```python
from build123d import *

# Parameters (mm, degrees)
F0_W     = 6
F0_H     = 6
F0_R     = 1.75
F2_DEPTH = 3
F1_W     = 9.8
F1_H     = 18
F3_DEPTH = 0.2


with BuildPart() as f2:
    # F0 (on Top) → F2 (new body)
    with BuildSketch(Plane.XY):
        with BuildLine():
            ThreePointArc((1.75, -6), (-1.237437, -4.762563), (0, -7.75))
            ThreePointArc((0, -7.75), (1.237437, -7.237437), (1.75, -6))
        make_face()
        Polygon((7.5, 9), (-7.5, 9), (-7.5, 3), (-7.5, -9), (0, -9), (7.5, -9), (7.5, 3), align=None)
        with BuildLine():
            ThreePointArc((1.75, -6), (1.237437, -7.237437), (0, -7.75))
            ThreePointArc((0, -7.75), (-1.237437, -4.762563), (1.75, -6))
        make_face(mode=Mode.SUBTRACT)
        with BuildLine():
            ThreePointArc((-8.75, 6), (-11.737437, 7.237437), (-10.5, 4.25))
            ThreePointArc((-10.5, 4.25), (-9.262563, 4.762563), (-8.75, 6))
        make_face()
        Polygon((-7.5, 3), (-7.5, 9), (-13.5, 9), (-13.5, 3), (-10.5, 3), align=None)
        with BuildLine():
            ThreePointArc((-8.75, 6), (-9.262563, 4.762563), (-10.5, 4.25))
            ThreePointArc((-10.5, 4.25), (-11.737437, 7.237437), (-8.75, 6))
        make_face(mode=Mode.SUBTRACT)
        with Locations((10.5, 6)):
            Rectangle(F0_W, F0_H)
        with Locations((10.5, 6)):
            Circle(F0_R, mode=Mode.SUBTRACT)
    extrude(amount=F2_DEPTH)

    # F1 (on face) → F3 (cut)
    with BuildSketch(Plane.XY):
        Rectangle(F1_W, F1_H)
    extrude(amount=F3_DEPTH, mode=Mode.SUBTRACT)


solid = f2.part
```
Build history of the part. All positions in model axes, mm. A direction names the side the tool comes from. Coordinates: 2 decimals unless noted, no trailing zeros. Order: outer loops, then holes, each group sorted by start corner. A loop starts at its lowest first (then second) coordinate and runs counter-clockwise, first axis right, second up. Notation, with made-up numbers: M -27,21.5 L 6,21.5 A18 ccw 6,34.5 Z; hole C 89.5,15.25 d11. An arc over 180 degrees is marked long. One line per question, with ' | ' between items. Start each with the question number.
1. Mould opens along Y. For faces 1 (the face through (11.31, 4.45, 1.48)), 2 (the face through (-7, 2, 0)), 3 (the face through (10, 3, 1)) say: +Y half, -Y half, draft (parallel to the pull), parting line (faces both ways), or undercut.
2. Cut at C-C (y = 1.5). Write the cut outline in (x, z), plus the area to 3 significant figures.
3. Cut at B-B (x = 10.5). Write the cut outline in (y, z), plus the area to 3 significant figures.
4. Cut at A-A (z = 2.2). Write the cut outline in (x, y), plus the area to 3 significant figures.
5. Tool access for faces 4 (the face through (0, 0, 0.2)), 5 (the face through (-11, 3, 1)), 6 (the face through (7.5, -3, 1)): list every direction of +Z, -Z, +X, -X, +Y, -Y with a clear straight run to the whole face (end or side of a thin tool).
6. Wall check: line 1 along Y through (x, z) = (10.5, 1.75); line 2 along Y through (x, z) = (0, 1); line 3 along X through (y, z) = (-6, 1.05). Give the ranges that are in metal, low to high. Write a range as [from, to].
7. Flat gauge pins, fed straight in: P1, Ø3, axis at x = -10.5, y = 6, coming from the -Z side; P2, Ø3, axis at x = -1, y = 0.5, coming from the -Z side; P3, Ø1.5, axis at x = -9, z = 2, coming from the -Y side; P4, Ø0.9, axis at y = -3, z = 1.5, coming from the -X side. Where does each tip first touch, or does it go through?
8. Cut at D-D (y = -6.5). Write the cut outline in (x, z).
The answers:
1) face 1: undercut | face 2: draft | face 3: -Y half
2) outline: M -7.5,0 L -4.9,0 L -4.9,0.2 L 4.9,0.2 L 4.9,0 L 7.5,0 L 7.5,3 L -7.5,3 Z | area: 43.0 mm2
3) outline: M 3,0 L 4.25,0 L 4.25,3 L 3,3 Z; M 7.75,0 L 9,0 L 9,3 L 7.75,3 Z | area: 7.50 mm2
4) outline: M -13.5,3 L -7.5,3 L -7.5,-9 L 7.5,-9 L 7.5,3 L 13.5,3 L 13.5,9 L -13.5,9 Z; hole C -10.5,6 d3.5; hole C 0,-6 d3.5; hole C 10.5,6 d3.5 | area: 313 mm2
5) face 4: -Z, +Y, -Y | face 5: +Z, -Z, -X, -Y | face 6: +Z, -Z, +X, -Y
6) line 1: y = [3, 4.25], [7.75, 9] | line 2: y = [-9, -7.75], [-4.25, 9] | line 3: x = [-7.5, -1.75], [1.75, 7.5]
7) P1: passes through | P2: stops at z = 0.2 | P3: stops at y = 3 | P4: stops at x = -7.5
8) outline: M -7.5,0 L -4.9,0 L -4.9,0.2 L -1.68,0.2 L -1.68,3 L -7.5,3 Z; M 1.68,0.2 L 4.9,0.2 L 4.9,0 L 7.5,0 L 7.5,3 L 1.68,3 Z
